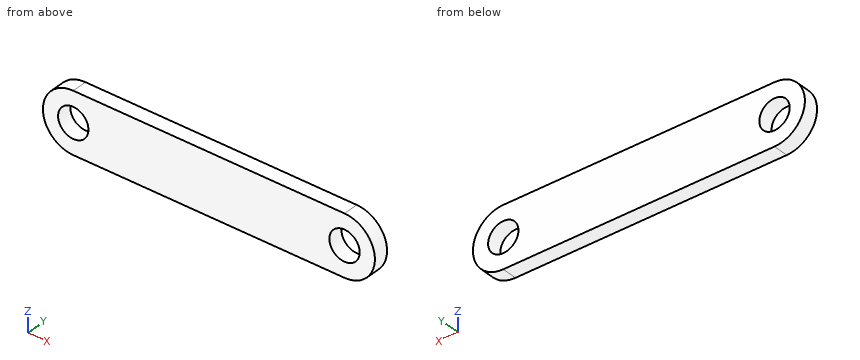
Autodesk Inventor part; units mm, degrees
ref_plane "YZ Plane" through (0, 0, 0) normal (1, 0, 0) x (0, 1, 0)
ref_plane "XZ Plane" through (0, 0, 0) normal (0, 1, 0) x (-1, 0, 0)
ref_plane "XY Plane" through (0, 0, 0) normal (0, 0, 1) x (1, 0, 0)
sketch "草圖3" plane through (0, 0, 0) normal (0, 1, 0) x (-1, 0, 0)
  line L0 (-99.36, 0) -> (10, 0) construction
  line L1 (-89.36, 10) -> (0, 10)
  line L2 (0, -10) -> (-89.36, -10)
  arc A0 (-89.36, 10) -> (-89.36, -10) centre (-89.36, 0) ccw
  arc A1 (0, -10) -> (0, 10) centre (0, 0) ccw
  circle A2 centre (-89.36, 0) radius 5
  circle A3 centre (0, 0) radius 5
  point P0 (-44.68, 0)
  dimension "hole" = 10
  dimension "d14" = 20
  dimension "center_distance" = 89.36
extrude "擠出3" add sketch "草圖3" along normal blind 5
equation "\"d14\" = 2 * hole"
properties part number "test6"
Read the model definition and answer for the solid it produces. Units are mm, in the model's axes. Coordinates: 2 decimals unless noted, no trailing zeros. Loops run counter-clockwise (first coordinate to the right, second up) from the corner with the lowest first, then second, coordinate; pieces in that order, holes last.
Q1. The part is cut by section C-C on z = -9. Write down the section's boundary in (x, y), and give its area (3 significant figures).
Q2. The part is cut by section A-A on z = 0. Write down the section's boundary in (x, y), and give its area (3 significant figures).
Q3. Consider probe 1 along Z at (x, y) = (89.36, 2.9); probe 2 along X at (y, z) = (4.55, -2); probe 3 along X at (y, z) = (4.05, -4.25). Determine where each line is inside the solid, lowest interval first.
Q4. This flat-tipped pin is pushed along its axis until it touches: pin 1 Ø1.5 at (y, z) = (4, -3) entering from -X. Where does it stop, or does it pass through?
Q5. The part is cut by section B-B on y = 2.55. Write down the section's boundary in (x, z).
Results below:
1. outline: (-4.36, 0) - (93.72, 0) - (93.72, 5) - (-4.36, 5) - close
1. area: 490 mm2
2. outline: (-10, 0) - (-5, 0) - (-5, 5) - (-10, 5) - close; (5, 0) - (84.36, 0) - (84.36, 5) - (5, 5) - close; (94.36, 0) - (99.36, 0) - (99.36, 5) - (94.36, 5) - close
2. area: 447 mm2
3. probe 1: z = -10 to -5, 5 to 10
3. probe 2: x = -9.8 to -4.58, 4.58 to 84.78, 93.94 to 99.16
3. probe 3: x = -9.05 to -2.63, 2.63 to 86.73, 91.99 to 98.41
4. pin 1: stops at x = -9.74
5. outline: (0, -10) - (89.36, -10) arc R10 ccw to (89.36, 10) - (0, 10) arc R10 ccw to start; hole circle Ø10 at (0, 0); hole circle Ø10 at (89.36, 0)
